Source: CAD feature listing. Evaluate the final solid. Frame: model axes, mm. Face numbers are marked on the shaded views. A direction names the side the tool comes from. Round coordinates to 2 decimals unless told otherwise and drop trailing zeros. Write each loop counter-clockwise with the first axis right and the second up, starting at its lowest first coordinate (ties: lowest second). Pieces come first, ordered by that corner, then holes. Notation, with made-up numbers: M 18,81 L 61,81 A12 ccw 61,97 Z; hole C -30.5,39 d8. An arc over 180 degrees is marked long. Answer in a Markdown table with one row per item.
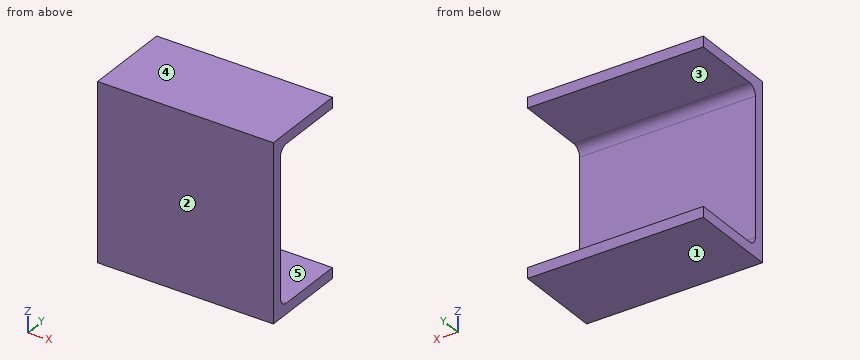
from build123d import *

# Parameters (mm, degrees)
BOSS_EXTRUDE1_DEPTH = 50.8


with BuildPart() as part:
    # Sketch1 → Boss-Extrude1 (new body)
    with BuildSketch(Plane(origin=(0, 0, 0), x_dir=(0, 0, -1), z_dir=(1, 0, 0))):
        with BuildLine():
            Line((-22.352, -7.112), (-22.352, 9.652))
            Line((-22.352, 9.652), (-22.352, 12.7))
            Line((-22.352, 12.7), (-25.4, 12.7))
            Line((-25.4, 12.7), (-25.4, -12.7))
            Line((-25.4, -12.7), (25.4, -12.7))
            Line((25.4, -12.7), (25.4, 12.7))
            Line((25.4, 12.7), (22.352, 12.7))
            Line((22.352, 12.7), (22.352, 9.652))
            Line((22.352, 9.652), (22.352, -7.112))
            ThreePointArc((22.352, -7.112), (21.608051224, -8.908051224), (19.812, -9.652))
            Line((19.812, -9.652), (-19.812, -9.652))
            ThreePointArc((-19.812, -9.652), (-21.608051224, -8.908051224), (-22.352, -7.112))
        make_face()
    extrude(amount=BOSS_EXTRUDE1_DEPTH)


solid = part.part
Q1. Section D-D (z = -18.5). Return loops of the section in (x, y), and give its area (3 significant figures).
Solutions:
| item | result |
|---|---|
| outline | M 0,-12.7 L 50.8,-12.7 L 50.8,-9.65 L 0,-9.65 Z |
| area | 155 mm2 |
Q2. Section C-C (y = -8.75). Return loops of the section in (x, z), and give its area (3 significant figures).
Solutions:
| item | result |
|---|---|
| outline | M 0,-25.4 L 50.8,-25.4 L 50.8,-21.75 L 0,-21.75 Z; M 0,21.75 L 50.8,21.75 L 50.8,25.4 L 0,25.4 Z |
| area | 371 mm2 |
Q3. Contact query for a flat-ended pin moving along its axis: pin 1 Ø1.5 at (x, z) = (37, -1.5) entering from +Y. Output: stop coordinate, or through.
Solutions:
| item | result |
|---|---|
| pin 1 | stops at y = -9.65 |
Q4. Section B-B (x = 13.5). Return loops of the section in (y, z), and give its area (3 significant figures).
Solutions:
| item | result |
|---|---|
| outline | M -12.7,-25.4 L 12.7,-25.4 L 12.7,-22.35 L -7.11,-22.35 A2.54 cw -9.65,-19.81 L -9.65,19.81 A2.54 cw -7.11,22.35 L 12.7,22.35 L 12.7,25.4 L -12.7,25.4 Z |
| area | 294 mm2 |
Q5. Material intervals for probe 1 along Z at (x, y) = (29.5, 7.25); probe 2 along Y at (x, z) = (27, -2); probe 3 along Z at (x, y) = (7, -7.5), sorted ascending.
Solutions:
| item | result |
|---|---|
| probe 1 | z = -25.4 to -22.35, 22.35 to 25.4 |
| probe 2 | y = -12.7 to -9.65 |
| probe 3 | z = -25.4 to -22.32, 22.32 to 25.4 |
Q6. Pull-direction query (Z, two-part tool) for the marked faces 1, 2 and 3; classes: pulls with the +Z half, pulls with the -Z half, needs draft (parallel to the pull), parting line crosses it, or undercut.
Solutions:
| item | result |
|---|---|
| face 1 | pulls with the -Z half |
| face 2 | needs draft |
| face 3 | undercut |
Q7. Access query for the marked faces 4 and 5. Directions: +Z, -Z, +X, -X, +Y, -Y. A direction counts if a zero-diameter tool reaches every point of the face in a straight line with its end or side. Return the directions, or none.
Solutions:
| item | result |
|---|---|
| face 4 | +Z, +X, -X, +Y, -Y |
| face 5 | +X, -X, +Y |
Q8. Section A-A (y = -3.25). Return loops of the section in (x, z), and give its area (3 significant figures).
Solutions:
| item | result |
|---|---|
| outline | M 0,-25.4 L 50.8,-25.4 L 50.8,-22.35 L 0,-22.35 Z; M 0,22.35 L 50.8,22.35 L 50.8,25.4 L 0,25.4 Z |
| area | 310 mm2 |
